Input: part model. Units: mm. Frame: model coordinates. Face numbers are marked on the shaded views. A direction names the side the tool comes from. Coordinates: 2 decimals unless noted, no trailing zeros. Order: outer loops, then holes, each group sorted by start corner. A loop starts at its lowest first (then second) coordinate and runs counter-clockwise, first axis right, second up. Notation, with made-up numbers: M 53,-27.5 L 88,-27.5 A12 cw 88,-23.5 Z; hole C 59,-32.75 d9. An arc over 180 degrees is marked long. One line per item, written item: value.
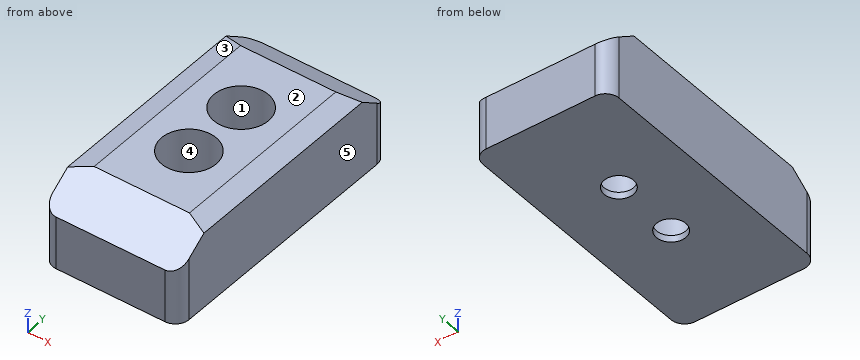
```python
from build123d import *

# Parameters (mm, degrees)
SKETCH1_W           = 20
SKETCH1_H           = 40
SKETCH1_R           = 2.15
BOSS_EXTRUDE1_DEPTH = 12
CHAMFER1_SIZE       = 3
CHAMFER1_SIZE2      = 0.803847577
CHAMFER2_SIZE       = 6
CHAMFER2_SIZE2      = 4.201245229
SKETCH2_R           = 4
CUT_EXTRUDE1_DEPTH  = 11
FILLET1_R           = 2


with BuildPart() as part:
    # Sketch1 → Boss-Extrude1 (new body)
    with BuildSketch(Plane.XY):
        Rectangle(SKETCH1_W, SKETCH1_H)
        with Locations((0, -5)):
            Circle(SKETCH1_R, mode=Mode.SUBTRACT)
        with Locations((0, 5)):
            Circle(SKETCH1_R, mode=Mode.SUBTRACT)
    extrude(amount=BOSS_EXTRUDE1_DEPTH)

    # Chamfer1
    chamfer1_edges = [part.edges().sort_by_distance(p)[0] for p in [
        (-10, 0, 12),
        (10, 0, 12),
    ]]
    chamfer1_side = [part.faces().sort_by_distance(p)[0] for p in [
        (0, 0, 12),
    ]]
    chamfer(chamfer1_edges, length=CHAMFER1_SIZE, length2=CHAMFER1_SIZE2, reference=chamfer1_side[0])

    # Chamfer2
    chamfer2_edges = [part.edges().sort_by_distance(p)[0] for p in [
        (0, -20, 12),
        (0, 20, 12),
    ]]
    chamfer2_side = [part.faces().sort_by_distance(p)[0] for p in [
        (0, 0, 12),
    ]]
    chamfer(chamfer2_edges, length=CHAMFER2_SIZE, length2=CHAMFER2_SIZE2, reference=chamfer2_side[0])

    # Sketch2 → Cut-Extrude1 (cut)
    with BuildSketch(Plane.XY.offset(12)):
        with Locations((0, 5)):
            Circle(SKETCH2_R)
        with Locations((0, -5)):
            Circle(SKETCH2_R)
    extrude(amount=-CUT_EXTRUDE1_DEPTH, mode=Mode.SUBTRACT)

    # Fillet1
    fillet1_edges = [part.edges().sort_by_distance(p)[0] for p in [
        (10, 20, 3.899377385),
        (10, -20, 3.899377385),
        (-10, -20, 3.899377385),
        (-10, 20, 3.899377385),
    ]]
    fillet(fillet1_edges, radius=FILLET1_R)


solid = part.part
```
(1) Access query for the marked faces 1 and 2. Directions: +Z, -Z, +X, -X, +Y, -Y. A direction counts if a zero-diameter tool reaches every point of the face in a straight line with its end or side. Return the directions, or none.
Data:
face 1: +Z
face 2: +Z, +X, -X, +Y, -Y
(2) Ray query, line 1 (Y direction, x = 0, z = 5); line 2 (X direction, y = -5, z = 0.5); line 3 (Y direction, x = 0, z = 0.85). Return the intervals inside material, ascending. Write a range as from..to.
Data:
line 1: y = -20..-9, -1..1, 9..20
line 2: x = -10..-2.15, 2.15..10
line 3: y = -20..-7.15, -2.85..2.85, 7.15..20
(3) First-contact query: pin 1 (10 mm diameter, centred on x = 4, y = 5.5, fed in from -Z); pin 2 (5 mm diameter, centred on x = 0, y = -5, fed in from +Z); pin 3 (3.5 mm diameter, centred on x = 0, y = 5, fed in from +Z). Flat tips, straight axial feed; report the tip coordinate or a pass-through.
Data:
pin 1: stops at z = 0
pin 2: stops at z = 1
pin 3: passes through
(4) Cut plane B-B on x = 0. Output: boundary loops of the cut face in (y, z).
Data:
outline: M -20,0 L -7.15,0 L -7.15,1 L -9,1 L -9,12 L -14,12 L -20,7.8 Z; M -2.85,0 L 2.85,0 L 2.85,1 L 1,1 L 1,12 L -1,12 L -1,1 L -2.85,1 Z; M 7.15,0 L 20,0 L 20,7.8 L 14,12 L 9,12 L 9,1 L 7.15,1 Z
(5) Cut plane D-D on y = -2. Output: boundary loops of the cut face in (x, z), plus the area to 3 significant figures.
Data:
outline: M -10,0 L 10,0 L 10,11.2 L 7,12 L 2.65,12 L 2.65,1 L -2.65,1 L -2.65,12 L -7,12 L -10,11.2 Z
area: 179 mm2
(6) Draft query along X for the marked faces 3, 4 and 5. Return one class per face: released by +X, released by -X, zero draft, split by the parting line, or undercut.
Data:
face 3: released by -X
face 4: undercut
face 5: released by +X
(7) Cut plane C-C on z = 6.75. Output: boundary loops of the cut face in (x, y).
Data:
outline: M -10,-18 A2 ccw -8,-20 L 8,-20 A2 ccw 10,-18 L 10,18 A2 ccw 8,20 L -8,20 A2 ccw -10,18 Z; hole C 0,-5 d8; hole C 0,5 d8
(8) Cut plane A-A on y = 5. Output: boundary loops of the cut face in (x, z).
Data:
outline: M -10,0 L -2.15,0 L -2.15,1 L -4,1 L -4,12 L -7,12 L -10,11.2 Z; M 2.15,0 L 10,0 L 10,11.2 L 7,12 L 4,12 L 4,1 L 2.15,1 Z
